from build123d import *

# Parameters (mm, degrees)
SKETCH_W     = 160
SKETCH_H     = 2300
PAD_DEPTH    = 30
PAD001_DEPTH = 11.45
SKETCH004_W  = 68
SKETCH004_H  = 45
PAD004_DEPTH = 13.945


with BuildPart() as part:
    # Sketch → Pad (new body)
    with BuildSketch(Plane.YZ):
        with Locations((-911.017, 830.848)):
            Rectangle(SKETCH_W, SKETCH_H)
    extrude(amount=PAD_DEPTH)

    # Sketch001 (on Face5 of Pad) → Pad001 (join)
    with BuildSketch(Plane(origin=(0, 0, 0), x_dir=(0, 1, 0), z_dir=(-1, 0, 0))):
        Polygon((-959.089896, 236.194146), (-863.09, 236.053045), (-863.159081, 189.053045), (-959.158977, 189.194146), align=None)
        Polygon((-959.09, -1851.352361), (-863.09, -1851.346955), (-863.087354, -1898.346955), (-959.087354, -1898.352361), align=None)
    extrude(amount=PAD001_DEPTH)

    # Sketch004 (on Face5 of Pad001) → Pad004 (join)
    with BuildSketch(Plane.YZ.offset(30)):
        with Locations((-881.01, -159.045)):
            Rectangle(SKETCH004_W, SKETCH004_H)
        with Locations((-881.01, 1785.955)):
            Rectangle(SKETCH004_W, SKETCH004_H)
    extrude(amount=PAD004_DEPTH)


with BuildPart() as part_1:
    # Body placement: moved
    add(part.part.moved(Location((103.004971, 1.762416, 16.745678))))


solid = part_1.part
Build history of the part. All positions in model axes, mm. Coordinates: 2 decimals unless noted, no trailing zeros. Order: outer loops, then holes, each group sorted by start corner. A loop starts at its lowest first (then second) coordinate and runs counter-clockwise, first axis right, second up. Notation, with made-up numbers: M 84.25,25.5 L 125.25,25.5 A24 ccw 125.25,62.5 Z; hole C 2,12.5 d1. An arc over 180 degrees is marked long. One line per question, with ' | ' between items. Start each with the question number.
Q1. Saw through at A-A (z = 1237). List the corners of the cut face in (x, y).
Q2. Flat gauge pins, fed straight in: pin 1 Ø4 at (x, y) = (143.5, -879) entering from -Z; pin 2 Ø2 at (y, z) = (-847, 1107.5) entering from -X (3 decimals); pin 3 Ø4 at (x, z) = (137.5, -137) entering from -Y. Where does each tip first touch, or does it go through?
Q3. Probe L1, parallel to Z at x = 138, y = -852.5; L2, parallel to Z at x = 100, y = -936; L3, parallel to X at y = -896, z = 1471.5. List the from-to ranges inside material, lowest first. Write a range as from..to.
Q4. Saw through at B-B (y = -880). List the corners of the cut face in (x, z).
Check values:
1) outline: M 103,-989.25 L 133,-989.25 L 133,-829.25 L 103,-829.25 Z
2) pin 1: stops at z = -164.8 | pin 2: stops at x = 103.005 | pin 3: stops at y = -913.25
3) L1: z = -164.8..-119.8, 1780.2..1825.2 | L2: z = -219.42..-172.42, 1868.1..1915.1 | L3: x = 103..133
4) outline: M 91.55,-219.33 L 103,-219.33 L 103,-302.41 L 133,-302.41 L 133,-164.8 L 146.95,-164.8 L 146.95,-119.8 L 133,-119.8 L 133,1780.2 L 146.95,1780.2 L 146.95,1825.2 L 133,1825.2 L 133,1997.59 L 103,1997.59 L 103,1915.09 L 91.55,1915.09 L 91.55,1868.09 L 103,1868.09 L 103,-172.33 L 91.55,-172.33 Z
